Read the model definition and answer for the solid it produces. Units are mm, in the model's axes. Face numbers are marked on the shaded views. A direction names the side the tool comes from. Coordinates: 2 decimals unless noted, no trailing zeros. Loops run counter-clockwise (first coordinate to the right, second up) from the corner with the lowest first, then second, coordinate; pieces in that order, holes last. Notation, with made-up numbers: (78.5, 16.25) - (84.5, 16.25) arc R23 cw to (84.5, 39.25) - close; hole circle Ø9 at (42, -4.5). An arc over 180 degrees is marked (long way). One line per item, written item: value. Start each with the question number.
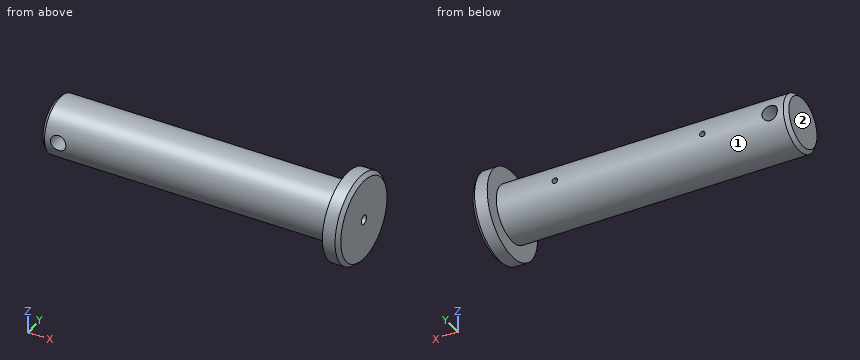
from build123d import *

# Parameters (mm, degrees)
ESBO_O2_R                  = 1.5
CORTE_EXTRUS_O1_DEPTH      = 92.370241873
CORTE_EXTRUS_O2_DEPTH      = 92.370241873
CORTE_EXTRUS_O2_DEPTH_BACK = 92.370241873
ESBO_O3_R                  = 4.25


with BuildPart() as part:
    # Esboço1 → Revolução1 (revolve)
    with BuildSketch(Plane.XY, mode=Mode.PRIVATE) as revolu_o1_sk:
        Polygon((84.69, 2.5), (84.69, 22.25), (82.69, 24.25), (75.69, 24.25), (75.69, 15.5), (-82.69, 15.5), (-84.69, 13.5), (-84.69, 0), (-44.69, 0), (-43.788709071, 1.5), (74.089139381, 1.5), (74.69, 2.5), align=None)
    revolve(revolu_o1_sk.sketch.rotate(Axis((-84.69, 0, 0), (1, 0, 0)), 90), axis=Axis((-84.69, 0, 0), (1, 0, 0)))

    # Esboço2 → Corte-extrusão1 (cut, through all)
    with BuildSketch(Plane(origin=(0, 0, 0), x_dir=(1, 0, 0), z_dir=(0, 1, 0))):
        with Locations(Location((43.39, 0, 0), (0, 0, 90))):
            Circle(ESBO_O2_R)
        with Locations(Location((-38.05, 0, 0), (0, 0, 90))):
            Circle(ESBO_O2_R)
    extrude(amount=CORTE_EXTRUS_O1_DEPTH, mode=Mode.SUBTRACT)

    # Esboço3 → Corte-extrusão2 (cut, two sides: drawn at the far end of the back side and taken through both)
    with BuildSketch(Plane(origin=(0, 0, 0), x_dir=(1, 0, 0), z_dir=(0, 1, 0)).offset(-CORTE_EXTRUS_O2_DEPTH_BACK)):
        with Locations(Location((-75.19, 0, 0), (0, 0, 270))):
            Circle(ESBO_O3_R)
    extrude(amount=CORTE_EXTRUS_O2_DEPTH + CORTE_EXTRUS_O2_DEPTH_BACK, mode=Mode.SUBTRACT)


solid = part.part
1) Section C-C, the plane x = -48.5 is taken. Determine the outline of the cut face in (y, z), and give its area (3 significant figures).
2) Straight lines are drawn through the part: L1, parallel to X at y = 11.75, z = 0; L2, parallel to Y at x = 19.5, z = 0; L3, parallel to X at y = 20, z = 2.5. For each, find the intervals that lie inside material, in ascending order.
3) For the marked faces 1 and 2, determine the directions among +Z, -Z, +X, -X, +Y, -Y from which every point of the face is accessible in a straight line to the end or side of a thin tool.
4) Section D-D, the plane x = 43.39 is taken. Determine the outline of the cut face in (y, z).
5) Section B-B, the plane x = -75.19 is taken. Determine the outline of the cut face in (y, z), and give its area (3 significant figures).
6) Flat-ended cylindrical pins translate along their axes: P1, Ø3, axis at x = 67.5, z = 3, coming from the -Y side; P2, Ø4, axis at y = 0, z = 0, coming from the +X side; P3, Ø1, axis at x = 30.5, z = -10.5, coming from the -Y side; P4, Ø5, axis at x = -75.19, z = 0, coming from the +Y side. Find the tip coordinate at first contact, or state that the pin passes through.
7) Section A-A, the plane x = 68 is taken. Determine the outline of the cut face in (y, z), and give its area (3 significant figures).
Answer below:
1. outline: circle Ø31 at (0, 0)
1. area: 755 mm2
2. L1: -84.69 to -79.44, -70.94 to -39.55, -36.55 to 41.89, 44.89 to 84.69
2. L2: -15.5 to -1.5, 1.5 to 15.5
2. L3: 75.69 to 84.69
3. face 1: -X
3. face 2: +Z, -Z, -X, +Y, -Y
4. outline: (0, -1.5) arc R1.5 cw to (0, 1.5) - (15.43, 1.5) arc R15.5 ccw (long way) to (15.43, -1.5) - close
5. outline: (-14.91, -4.25) arc R15.5 ccw to (14.91, -4.25) - close; (-14.91, 4.25) - (14.91, 4.25) arc R15.5 ccw to start
5. area: 495 mm2
6. P1: y = -15.43
6. P2: x = 74.39
6. P3: y = -11.84
6. P4: through
7. outline: circle Ø31 at (0, 0); hole circle Ø3 at (0, 0)
7. area: 748 mm2
